Model file for the job. Use its own axes, mm. Coordinates: 2 decimals unless noted, no trailing zeros. Loops run counter-clockwise (first coordinate to the right, second up) from the corner with the lowest first, then second, coordinate; pieces in that order, holes last. Notation, with made-up numbers: (66, -8) -> (117, -8) arc R30 cw to (117, 20) -> close; hole circle Ø10 at (52.25, -26). An arc over 180 degrees is marked (long way). Use one line per item in the form item = value.
```python
from build123d import *

# Parameters (mm, degrees)
F0_R     = 7.9375
F0_R_2   = 12.7
F1_DEPTH = 3.175


# Not quite as in the source:
# - a length typed as a fraction of an inch, garbled in the dataset ("3 / 203.2 mm" for 3/8 in), is restored


with BuildPart() as f1:
    # F0 (on Right) → F1 (new body)
    with BuildSketch(Plane.YZ):
        with BuildLine():
            Line((35.9976727843, 33.7128622103), (-11.5086332291, 33.7128622103))
            ThreePointArc((-11.5086332291, 33.7128622103), (-20.4888893502, 29.9931183314), (-24.2086332291, 21.0128622103))
            Line((-24.2086332291, 21.0128622103), (-24.2086332291, 14.6628622103))
            ThreePointArc((-24.2086332291, 14.6628622103), (-20.4888893502, 5.6826060893), (-11.5086332291, 1.9628622103))
            Line((-11.5086332291, 1.9628622103), (35.9976727843, 1.9628622103))
            ThreePointArc((35.9976727843, 1.9628622103), (44.9779289054, 5.6826060893), (48.6976727843, 14.6628622103))
            Line((48.6976727843, 14.6628622103), (48.6976727843, 21.0128622103))
            ThreePointArc((48.6976727843, 21.0128622103), (44.9779289054, 29.9931183314), (35.9976727843, 33.7128622103))
        make_face()
        with Locations((-7.3484922707, 16.9180016965)):
            Circle(F0_R, mode=Mode.SUBTRACT)
        with Locations((30.7515077293, 17.8526993841)):
            Circle(F0_R_2, mode=Mode.SUBTRACT)
    extrude(amount=F1_DEPTH)


solid = f1.part
```
Q1. Band-saw the part on A-A, the plane y = 23. Write the cut outline in (x, z) (3 decimals), and give its area (3 significant figures).
Result:
outline = (0, 1.963) -> (3.175, 1.963) -> (3.175, 7.793) -> (0, 7.793) -> close; (0, 27.913) -> (3.175, 27.913) -> (3.175, 33.713) -> (0, 33.713) -> close
area = 36.9 mm2
Q2. Band-saw the part on D-D, the plane z = 20. Write the cut outline in (x, y) (3 decimals).
Result:
outline = (0, -24.209) -> (3.175, -24.209) -> (3.175, -14.663) -> (0, -14.663) -> close; (0, -0.034) -> (3.175, -0.034) -> (3.175, 18.234) -> (0, 18.234) -> close; (0, 43.269) -> (3.175, 43.269) -> (3.175, 48.698) -> (0, 48.698) -> close
Q3. Band-saw the part on C-C, the plane x = 2.3. Write the cut outline in (y, z) (1 decimal).
Result:
outline = (-24.2, 14.7) arc R12.7 ccw to (-11.5, 2) -> (36, 2) arc R12.7 ccw to (48.7, 14.7) -> (48.7, 21) arc R12.7 ccw to (36, 33.7) -> (-11.5, 33.7) arc R12.7 ccw to (-24.2, 21) -> close; hole circle Ø15.9 at (-7.3, 16.9); hole circle Ø25.4 at (30.8, 17.9)
Q4. Mould opens along Z. For faces 1 (the face through (3.175, 12, 18)), 2 (the face through (1.565, 42.865, 21.667)), 3 (the face through (1.57, -9.07, 9.17)), 4 (the face through (2, 13, 33.713)) say: released by +Z, released by -Z, zero draft, split by the parting line, or undercut.
Result:
face_1 = zero draft
face_2 = undercut
face_3 = undercut
face_4 = released by +Z
Q5. Wall check: line 1 along Y through (x, z) = (1.7, 21); line 2 along Y through (x, z) = (2.4, 13); line 3 along Z through (x, y) = (1.4, 32). Give the ranges that are in metal, low to high.
Result:
line_1 = -24.21 to -14.16, -0.54 to 18.45, 43.06 to 48.7
line_2 = -24.1 to -14.25, -0.45 to 19.02, 42.49 to 48.59
line_3 = 1.96 to 5.21, 30.49 to 33.71
Q6. Band-saw the part on B-B, the plane z = 27.5. Write the cut outline in (x, y) (3 decimals), and give its area (3 significant figures).
Result:
outline = (0, -22.427) -> (3.175, -22.427) -> (3.175, 22.492) -> (0, 22.492) -> close; (0, 39.011) -> (3.175, 39.011) -> (3.175, 46.916) -> (0, 46.916) -> close
area = 168 mm2
